Geometry: final body of the model. Coordinates: model frame, mm. Face numbers are marked on the shaded views. A direction names the side the tool comes from. Give positions to 0.01 mm unless a question says otherwise; leave off trailing zeros. Write each loop counter-clockwise with the first axis right and the second up, starting at its lowest first coordinate (ties: lowest second). Pieces come first, ordered by that corner, then holes. Notation, with made-up numbers: (-40, -35.5) -> (-13, -35.5) arc R14 ccw to (-13, -20.5) -> close; hole circle Ø2 at (28, -16.5). An arc over 180 degrees is marked (long way). Use CSV: the item, a comma, the result in double quotes. Start each with the question number.
1) Contact query for flat-ended pins moving along their axis: P1, Ø6.5, axis at x = 3, z = 16.5, coming from the -Y side; P2, Ø6.5, axis at x = 3, y = 8, coming from the +Z side; P3, Ø4, axis at x = 0, z = 15.9, coming from the +Y side. Output: stop coordinate, or through.
2) Material intervals for line 1 (Y direction, x = 3, z = 19); line 2 (Z direction, x = 0.5, y = 111.5); line 3 (Z direction, x = -2.5, y = 105), sorted ascending. Write a range as [from, to].
3) Set-up query: the marked faces 1 and 2. Return all of +Z, -Z, +X, -X, +Y, -Y with unobstructed straight access to the full face (end or side cutting, diameter ignored); none if empty.
4) Section A-A (z = 14.75). Count the separate pieces of the cut face and the enclosed holes in it, plus the area to 3 significant figures.
5) Section C-C (y = 113). Output: boundary loops of the cut face in (x, z) (3 decimals).
6) Section B-B (z = -2.5). Output: boundary loops of the cut face in (x, y).
```python
from build123d import *

# Parameters (mm, degrees)
SKETCH2_R           = 6.35
SKETCH2_R_2         = 4.445
BOSS_EXTRUDE1_DEPTH = 127
BOSS_EXTRUDE2_START = -127
SKETCH3_R           = 2.54
BOSS_EXTRUDE2_DEPTH = 127
SKETCH4_W           = 31.75
SKETCH4_H           = 6.4008
SKETCH4_H_2         = 12.7
CUT_EXTRUDE1_DEPTH  = 127


with BuildPart() as part:
    # Sketch2 → Boss-Extrude1 (new body)
    with BuildSketch(Plane(origin=(0, 0, 0), x_dir=(1, 0, 0), z_dir=(0, 1, 0))):
        with Locations(Location((0, 0, 0), (0, 0, 270))):
            Circle(SKETCH2_R)
        with Locations(Location((0, 0, 0), (0, 0, 270))):
            Circle(SKETCH2_R_2, mode=Mode.SUBTRACT)
    extrude(amount=BOSS_EXTRUDE1_DEPTH)

    # Sketch3 → Boss-Extrude2 (add)
    with BuildSketch(Plane(origin=(0, 127, 0), x_dir=(1, 0, 0), z_dir=(0, 1, 0)).offset(BOSS_EXTRUDE2_START)):
        with BuildLine():
            Line((-6.35, 0), (-6.35, -15.898089304))
            ThreePointArc((-6.35, -15.898089304), (0, -22.248089304), (6.35, -15.898089304))
            Line((6.35, -15.898089304), (6.35, 0))
            ThreePointArc((6.35, 0), (0, -6.35), (-6.35, 0))
        make_face()
        with Locations(Location((0, -15.898089304, 0), (0, 0, 270))):
            Circle(SKETCH3_R, mode=Mode.SUBTRACT)
    extrude(amount=BOSS_EXTRUDE2_DEPTH)

    # Sketch4 → Cut-Extrude1 (cut)
    with BuildSketch(Plane(origin=(6.35, 0, 0), x_dir=(0, 0, -1), z_dir=(1, 0, 0))):
        with Locations((-21.613089304, 28.6004)):
            Rectangle(SKETCH4_W, SKETCH4_H)
        with Locations((-21.613089304, 66.7004)):
            Rectangle(SKETCH4_W, SKETCH4_H)
        with Locations((-21.613089304, 104.8004)):
            Rectangle(SKETCH4_W, SKETCH4_H)
        with Locations((-21.613089304, 6.35)):
            Rectangle(SKETCH4_W, SKETCH4_H_2)
    extrude(amount=-CUT_EXTRUDE1_DEPTH, mode=Mode.SUBTRACT)


solid = part.part
```
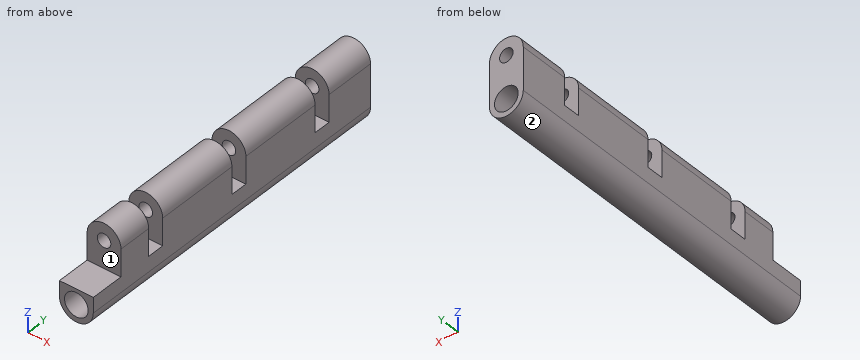
Answers follow:
1,P1,"stops at y = 12.7"
1,P2,"stops at z = 5.74"
1,P3,"passes through"
2,line 1,"y = [12.7, 25.4], [31.8, 63.5], [69.9, 101.6], [108, 127]"
2,line 2,"z = [-6.33, -4.42], [4.42, 13.41], [18.39, 22.23]"
2,line 3,"z = [-5.84, -3.68], [3.68, 5.74]"
3,face 1,"+Z, +X, -X, -Y"
3,face 2,"-Z, +Y, -Y"
4,separate pieces,"8"
4,enclosed holes,"0"
4,area,"777 mm^2"
5,outline,"(-6.35, 0) arc R6.35 ccw to (6.35, 0) -> (6.35, 15.898) arc R6.35 ccw to (-6.35, 15.898) -> close; hole circle Ø8.89 at (0, 0); hole circle Ø5.08 at (0, 15.898)"
6,outline,"(-5.84, 0) -> (-3.68, 0) -> (-3.68, 127) -> (-5.84, 127) -> close; (3.68, 0) -> (5.84, 0) -> (5.84, 127) -> (3.68, 127) -> close"
